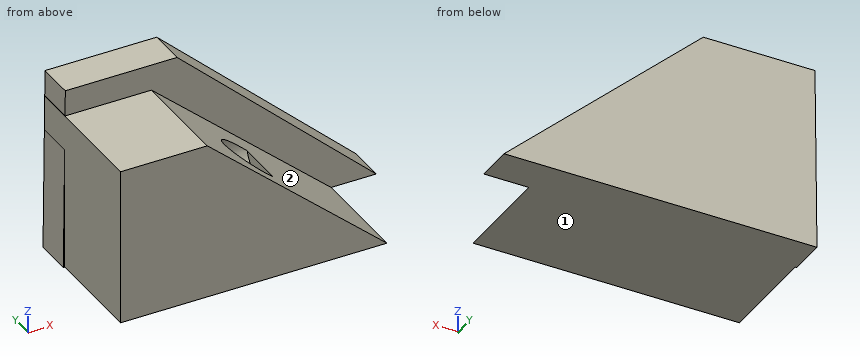
```python
from build123d import *

# Parameters (mm, degrees)
F1_DEPTH = 10.16
F3_DEPTH = 38.1
F4_R     = 6.858397
F5_DEPTH = 25.4


with BuildPart() as f1:
    # F0 (on Front) → F1 (new body)
    with BuildSketch(Plane.XZ):
        Polygon((-13.918791, 33.829112), (-44.521693, 33.829112), (-45.074757, -16.684113), (40.650241, -16.684113), align=None)
    extrude(amount=F1_DEPTH)

    # F2 (on Front) → F3 (join)
    with BuildSketch(Plane.XZ):
        Polygon((-20.924274, 26.639275), (-44.70605, 26.639275), (-44.70605, -16.684113), (28.298469, -16.684113), align=None)
    extrude(amount=F3_DEPTH)

    # F4 (on Right) → F5 (cut)
    with BuildSketch(Plane.YZ):
        with Locations((-26.45492, 10.047339)):
            Circle(F4_R)
    extrude(amount=-F5_DEPTH, mode=Mode.SUBTRACT)


solid = f1.part
```
Check sheet for the modelled part. Datum: model origin and axes. Units: mm. Face numbers are marked on the shaded views. A direction names the side the tool comes from. Round coordinates to 2 decimals unless told otherwise and drop trailing zeros. Loops run counter-clockwise (first coordinate to the right, second up) from the corner with the lowest first, then second, coordinate; pieces in that order, holes last. Notation, with made-up numbers: (61, -25) - (74, -25) arc R17 ccw to (74, -6) - close; hole circle Ø1 at (-30.5, 21). An arc over 180 degrees is marked (long way). Write item = value, one per line. Start each with the question number.
Q1. Section check A-A (y = -5.5). Record the boundary of the cut face in (x, z).
Q2. Thickness scan on L1, parallel to Z at x = -32.5, y = -12; L2, parallel to X at y = -9, z = 18; L3, parallel to Z at x = -23, y = -20.5. Record the ranges inside material, lowest first.
Q3. Section check C-C (z = -5.5). Record the boundary of the cut face in (x, y), plus the area to 3 significant figures.
Q4. Section check D-D (y = -26). Record the boundary of the cut face in (x, z), plus the area to 3 significant figures.
Q5. Section check B-B (x = -30.5). Record the boundary of the cut face in (y, z), plus the area to 3 significant figures.
Q6. Depth check by flat-ended pin: P1, Ø12, axis at y = -15.5, z = 10.5, coming from the -X side; P2, Ø19, axis at y = -21, z = 4.5, coming from the -X side; P3, Ø11, axis at y = -29.5, z = 10.5, coming from the +X side. Enter the tip coordinate at first touch or a pass-through.
Q7. Access from +Z, -Z, +X, -X, +Y, -Y to the whole of each face (thin tool, end or side, straight path). Record for the marked faces 1 and 2.
Derived:
q1.outline = (-45.07, -16.68) - (40.65, -16.68) - (-13.92, 33.83) - (-44.52, 33.83) - (-44.6, 26.64) - (-44.71, 26.64) - (-44.71, 16.99) - close
q2.L1 = -16.68 to 26.64
q2.L2 = -44.71 to 3.18
q2.L3 = -16.68 to 6.64, 13.45 to 26.64
q3.outline = (-44.95, -10.16) - (-44.71, -10.16) - (-44.71, -38.1) - (15.59, -38.1) - (15.59, -10.16) - (28.57, -10.16) - (28.57, 0) - (-44.95, 0) - close
q3.area = 2,430 mm^2
q4.outline = (-44.71, -16.68) - (28.3, -16.68) - (0, 8.22) - (0, 3.2) - (-25.4, 3.2) - (-25.4, 16.89) - (-9.85, 16.89) - (-20.92, 26.64) - (-44.71, 26.64) - close
q4.area = 1,790 mm^2
q5.outline = (-38.1, -16.68) - (0, -16.68) - (0, 33.83) - (-10.16, 33.83) - (-10.16, 26.64) - (-38.1, 26.64) - close
q5.area = 1,720 mm^2
q6.P1 = -44.81
q6.P2 = -44.71
q6.P3 = 3.66
q7.face_1 = -Z, +X, -X, +Y, -Y
q7.face_2 = +Z, +X, -Y
